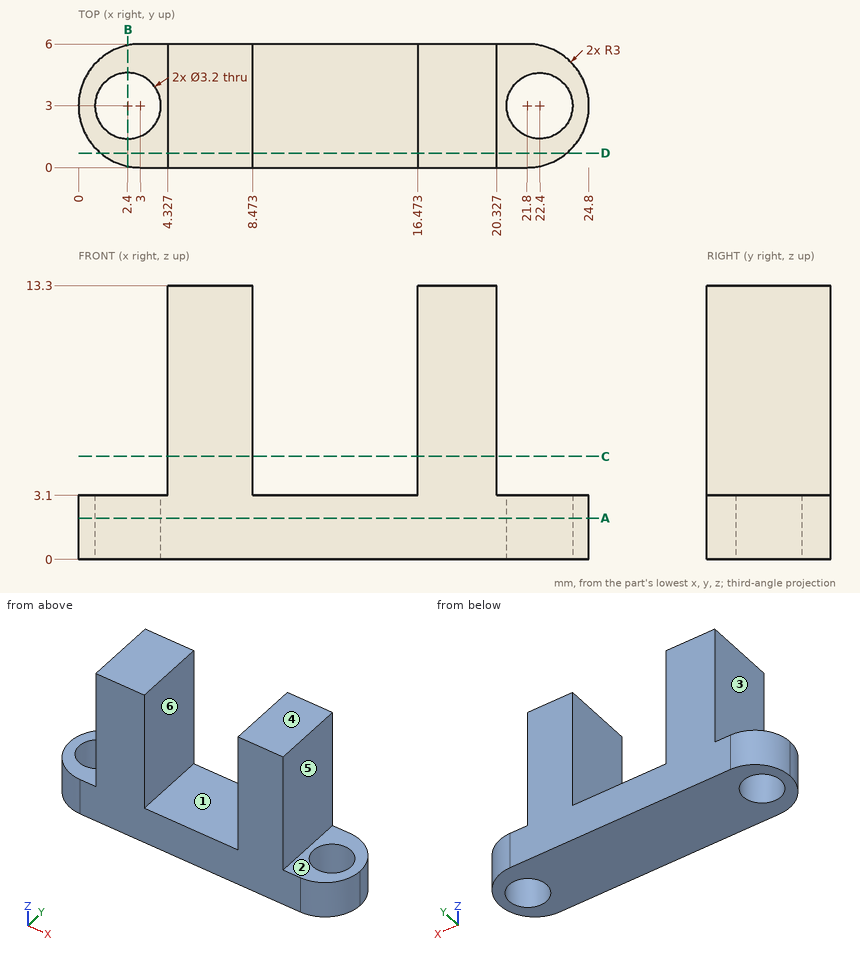
Input: dimensioned drawing with shaded views. Units: mm. Origin: part minimum x, y, z. A direction names the side the tool comes from. Round coordinates to 2 decimals unless told otherwise and drop trailing zeros. Order: outer loops, then holes, each group sorted by start corner. A loop starts at its lowest first (then second) coordinate and runs counter-clockwise, first axis right, second up. Notation, with made-up numbers: (89, -17.75) -> (135, -17.75) arc R6 cw to (135, -10.75) -> close; hole circle Ø4 at (-4, 86). An arc over 180 degrees is marked (long way). Put each result on its own line as item: value. Start each with the question number.
Q1. Section B-B on x = 2.4. Return the cut outline in (y, z).
Q2. Reachability of the marked faces 4, 5 and 6 from +Z, -Z, +X, -X, +Y, -Y: full face, straight path, thin tool, end or side. Return the list, or none.
Q3. Pull-direction query (X, two-part tool) for the marked faces 1, 2 and 3; classes: +X half, -X half, draft (parallel to the pull), parting line (faces both ways), or undercut.
Q4. Section C-C on z = 5. Return the cut outline in (x, y), and give its area (3 significant figures).
Q5. First-contact query: pin 1 (1.3 mm diameter, centred on x = 22, y = 3, fed in from +Z); pin 2 (1.8 mm diameter, centred on y = 4, z = 7, fed in from -X); pin 3 (2 mm diameter, centred on x = 18, z = 10, fed in from -Y); pin 4 (3 mm diameter, centred on y = 3.5, z = 8.5, fed in from +X). Flat tips, straight axial feed; report the tip coordinate or a pass-through.
Q6. Line query: probe 1 along X at (y, z) = (2.8, 5.25); probe 2 along X at (y, z) = (2.4, 2.5); probe 3 along Z at (x, y) = (10.75, 0.6). Output: solid intervals per line, ascending.
Q7. Section D-D on y = 0.7. Return the cut outline in (x, z), and give its area (3 significant figures).
Q8. Section A-A on z = 2. Return the cut outline in (x, y).
Ans:
1. outline: (0.06, 0) -> (1.4, 0) -> (1.4, 3.1) -> (0.06, 3.1) -> close; (4.6, 0) -> (5.94, 0) -> (5.94, 3.1) -> (4.6, 3.1) -> close
2. face 4: +Z, +X, -X, +Y, -Y
2. face 5: +Z, +X, +Y, -Y
2. face 6: +Z, +Y, -Y
3. face 1: undercut
3. face 2: draft
3. face 3: -X half
4. outline: (4.33, 0) -> (8.47, 0) -> (8.47, 6) -> (4.33, 6) -> close; (16.47, 0) -> (20.33, 0) -> (20.33, 6) -> (16.47, 6) -> close
4. area: 48.0 mm2
5. pin 1: passes through
5. pin 2: stops at x = 4.33
5. pin 3: stops at y = 0
5. pin 4: stops at x = 20.33
6. probe 1: x = 4.33 to 8.47, 16.47 to 20.33
6. probe 2: x = 0.06 to 0.92, 3.88 to 20.92, 23.88 to 24.74
6. probe 3: z = 0 to 3.1
7. outline: (1.07, 0) -> (23.73, 0) -> (23.73, 3.1) -> (20.33, 3.1) -> (20.33, 13.3) -> (16.47, 13.3) -> (16.47, 3.1) -> (8.47, 3.1) -> (8.47, 13.3) -> (4.33, 13.3) -> (4.33, 3.1) -> (1.07, 3.1) -> close
7. area: 152 mm2
8. outline: (3, 0) -> (21.8, 0) arc R3 ccw to (21.8, 6) -> (3, 6) arc R3 ccw to start; hole circle Ø3.2 at (2.4, 3); hole circle Ø3.2 at (22.4, 3)
